from build123d import *

# Parameters (mm, degrees)
F1_DEPTH = 425


with BuildPart() as f1:
    # F0 (on Right) → F1 (new body, symmetric)
    with BuildSketch(Plane.YZ):
        with BuildLine():
            Line((75, -9.5), (75, 0))
            Line((75, 0), (0, 0))
            Line((0, 0), (0, -150))
            Line((0, -150), (75, -150))
            Line((75, -150), (75, -140.5))
            Line((75, -140.5), (16, -140.5))
            ThreePointArc((16, -140.5), (8.928932, -137.571068), (6, -130.5))
            Line((6, -130.5), (6, -19.5))
            ThreePointArc((6, -19.5), (8.928932, -12.428932), (16, -9.5))
            Line((16, -9.5), (75, -9.5))
        make_face()
    extrude(amount=F1_DEPTH, both=True)


solid = f1.part
Read the model definition and answer for the solid it produces. Units are mm, in the model's axes. A direction names the side the tool comes from. Round coordinates to 2 decimals unless told otherwise and drop trailing zeros. Order: outer loops, then holes, each group sorted by start corner. A loop starts at its lowest first (then second) coordinate and runs counter-clockwise, first axis right, second up.
1) The part is cut by section A-A on y = 47.5. Write down the section's boundary in (x, z).
2) The mould has two halves that part along Z. Classify faces 1 (the face through (6, 0, -74)), 2 (the face through (6, 6, -76)), 3 (the face through (6, 38, 0)): released by +Z, released by -Z, zero draft, split by the parting line, or undercut.
3) For faces 4 (the face through (6, 46, -140.5)), 5 (the face through (425, 4, -75)), determine the directions among +Z, -Z, +X, -X, +Y, -Y from which every point of the face is accessible in a straight line to the end or side of a thin tool.
4) The part is cut by section B-B on x = -56. Write down the section's boundary in (y, z).
5) The part is cut by section C-C on z = -105.5. Write down the section's boundary in (x, y).
6) A flat-ended cylindrical pin translates along its axis: pin 1 (1.5 mm diameter, centred on x = 5, z = -19.5, fed in from +Y). Find the tip coordinate at first contact, or state that the pin passes through.
7) Straight lines are drawn through the part: L1, parallel to Z at x = 1, y = 46; L2, parallel to Y at x = 348, z = -130; L3, parallel to Z at x = 47.5, y = 13.5. For each, find the intervals that lie inside material, in ascending order.
Resolved:
1. outline: (-425, -150) - (425, -150) - (425, -140.5) - (-425, -140.5) - close; (-425, -9.5) - (425, -9.5) - (425, 0) - (-425, 0) - close
2. face 1: zero draft
2. face 2: undercut
2. face 3: released by +Z
3. face 4: +X, -X, +Y
3. face 5: +Z, -Z, +X, +Y, -Y
4. outline: (0, -150) - (75, -150) - (75, -140.5) - (16, -140.5) arc R10 cw to (6, -130.5) - (6, -19.5) arc R10 cw to (16, -9.5) - (75, -9.5) - (75, 0) - (0, 0) - close
5. outline: (-425, 0) - (425, 0) - (425, 6) - (-425, 6) - close
6. pin 1: stops at y = 6.03
7. L1: z = -150 to -140.5, -9.5 to 0
7. L2: y = 0 to 6
7. L3: z = -150 to -140.18, -9.82 to 0
